from build123d import *

# Parameters (mm, degrees)
F0_R     = 2.75
F1_DEPTH = 36.8
F2_R     = 3.2
F2_R_2   = 12.15
F3_DEPTH = 12.5
F4_W     = 7
F4_H     = 7
F5_DEPTH = 25


with BuildPart() as f1:
    # F0 (on Top) → F1 (new body)
    with BuildSketch(Plane.XY):
        with BuildLine():
            ThreePointArc((-11.5987953556, -1.3), (-11.4499860347, -0.657556004), (-11.4, 0))
            ThreePointArc((-11.4, 0), (-11.4499860347, 0.657556004), (-11.5987953556, 1.3))
            Line((-11.5987953556, 1.3), (-13, 1.3))
            Line((-13, 1.3), (-13, 0))
            Line((-13, 0), (-13, -1.3))
            Line((-13, -1.3), (-11.5987953556, -1.3))
        make_face()
        with BuildLine():
            ThreePointArc((-11.5987953556, 1.3), (-11.4499860347, 0.657556004), (-11.4, 0))
            ThreePointArc((-11.4, 0), (-11.4499860347, -0.657556004), (-11.5987953556, -1.3))
            Line((-11.5987953556, -1.3), (11.5987953556, -1.3))
            ThreePointArc((11.5987953556, -1.3), (11.4, 0), (11.5987953556, 1.3))
            Line((11.5987953556, 1.3), (-11.5987953556, 1.3))
        make_face()
        with BuildLine():
            Line((-13, 1.3), (-11.5987953556, 1.3))
            ThreePointArc((-11.5987953556, 1.3), (-20.1, 0), (-11.5987953556, -1.3))
            Line((-11.5987953556, -1.3), (-13, -1.3))
            Line((-13, -1.3), (-13, 0))
            Line((-13, 0), (-13, 1.3))
        make_face()
        with Locations((-15.75, 0)):
            Circle(F0_R, mode=Mode.SUBTRACT)
        with BuildLine():
            Line((13, 1.3), (11.5987953556, 1.3))
            ThreePointArc((11.5987953556, 1.3), (11.4, 0), (11.5987953556, -1.3))
            Line((11.5987953556, -1.3), (13, -1.3))
            Line((13, -1.3), (13, 0))
            Line((13, 0), (13, 1.3))
        make_face()
        with BuildLine():
            ThreePointArc((20.1, 0), (16.407556004, 4.3000139653), (11.5987953556, 1.3))
            Line((11.5987953556, 1.3), (13, 1.3))
            Line((13, 1.3), (13, 0))
            Line((13, 0), (13, -1.3))
            Line((13, -1.3), (11.5987953556, -1.3))
            ThreePointArc((11.5987953556, -1.3), (16.407556004, -4.3000139653), (20.1, 0))
        make_face()
        with BuildLine():
            ThreePointArc((18.5, 0), (15.75, -2.75), (13, 0))
            ThreePointArc((13, 0), (15.75, 2.75), (18.5, 0))
        make_face(mode=Mode.SUBTRACT)
    extrude(amount=F1_DEPTH)

    # F2 (on Front) → F3 (cut, symmetric)
    with BuildSketch(Plane.XZ):
        with Locations((0, 18.4)):
            Circle(F2_R)
        Circle(F2_R_2)
        with Locations((0, 36.8)):
            Circle(F2_R_2)
    extrude(amount=F3_DEPTH, both=True, mode=Mode.SUBTRACT)

    # F4 (on Front) → F5 (cut)
    with BuildSketch(Plane.XZ):
        with Locations((0, 18.4)):
            Rectangle(F4_W, F4_H)
    extrude(amount=-F5_DEPTH, mode=Mode.SUBTRACT)


solid = f1.part
Geometry check sheet. Reference: the model listing, model coordinates, mm. A direction names the side the tool comes from. Coordinates: 2 decimals unless noted, no trailing zeros. Order: outer loops, then holes, each group sorted by start corner. A loop starts at its lowest first (then second) coordinate and runs counter-clockwise, first axis right, second up. Notation, with made-up numbers: (49.25, -16.75) -> (103.25, -16.75) arc R17 ccw to (103.25, -7.75) -> close; hole circle Ø7 at (67, -19). An arc over 180 degrees is marked (long way). Use a Markdown table: item, result. Add a question column.
1. Cross-section at D-D (x = 0). Enter the section's corners in (y, z), and give its area (3 significant figures).
2. Cross-section at C-C (y = -3.5). Enter the section's corners in (x, z).
3. Material ranges on L1, parallel to X at y = 0.25, z = 15.5; L2, parallel to Y at x = -15.75, z = 26; L3, parallel to X at y = -1.25, z = 33, recorded low to high.
4. Mould release check, pull along Y, two halves, no side actions. Record for faces 4 (the face through (0, -1.3, 15)), 5 (the face through (-20.097, 0.173, 18.142)), 6 (the face through (-18.5, 0.1, 18.1)), 7 (the face through (-3.5, 1, 18)): pulls with the +Y half, pulls with the -Y half, needs draft (parallel to the pull), parting line crosses it, or undercut.
5. Set-up check for faces 1 (the face through (0, 1, 21.9)), 2 (the face through (-5, 1.3, 18)), 3 (the face through (-0.267, -0.034, 24.653)): record each of +Z, -Z, +X, -X, +Y, -Y from which the full face is reachable in a straight line by a thin tool's end or side.
6. Go/stop test with flat-tipped pins: pin 1 Ø5 at (x, y) = (-7.5, 1.5) entering from -Z; pin 2 Ø0.6 at (x, y) = (0, 1) entering from -Z; pin 3 Ø1 at (x, z) = (9.5, 14.5) entering from -Y. Record where each tip stops, or that it passes through.
7. Cross-section at A-A (z = 18.4). Enter the section's corners in (x, y).
8. Cross-section at B-B (x = -15.75). Enter the section's corners in (y, z), and give its area (3 significant figures).
Filled sheet:
| question | item | result |
|---|---|---|
| 1 | outline | (-1.3, 12.15) -> (1.3, 12.15) -> (1.3, 14.9) -> (0, 14.9) -> (0, 15.2) -> (-1.3, 15.2) -> close; (-1.3, 21.6) -> (0, 21.6) -> (0, 21.9) -> (1.3, 21.9) -> (1.3, 24.65) -> (-1.3, 24.65) -> close |
| 1 | area | 15.1 mm2 |
| 2 | outline | (-18.33, 0) -> (-13.17, 0) -> (-13.17, 36.8) -> (-18.33, 36.8) -> close; (13.17, 0) -> (18.33, 0) -> (18.33, 36.8) -> (13.17, 36.8) -> close |
| 3 | L1 | -20.09 to -18.49, -13.01 to -3.5, 3.5 to 13.01, 18.49 to 20.09 |
| 3 | L2 | -4.35 to -2.75, 2.75 to 4.35 |
| 3 | L3 | -19.92 to -18.2, -13.3 to -11.54, 11.54 to 13.3, 18.2 to 19.92 |
| 4 | face 4 | pulls with the -Y half |
| 4 | face 5 | parting line crosses it |
| 4 | face 6 | undercut |
| 4 | face 7 | needs draft |
| 5 | face 1 | +Y |
| 5 | face 2 | +Z, -Z, +Y |
| 5 | face 3 | +Z, +Y, -Y |
| 6 | pin 1 | z = 6.91 |
| 6 | pin 2 | z = 12.15 |
| 6 | pin 3 | y = -1.3 |
| 7 | outline | (-11.6, -1.3) -> (-3.2, -1.3) -> (-3.2, 0) -> (-3.5, 0) -> (-3.5, 1.3) -> (-11.6, 1.3) arc R4.35 ccw (long way) to start; (3.2, -1.3) -> (11.6, -1.3) arc R4.35 ccw (long way) to (11.6, 1.3) -> (3.5, 1.3) -> (3.5, 0) -> (3.2, 0) -> close; hole circle Ø5.5 at (-15.75, 0); hole circle Ø5.5 at (15.75, 0) |
| 8 | outline | (-4.35, 0) -> (-2.75, 0) -> (-2.75, 36.8) -> (-4.35, 36.8) -> close; (2.75, 0) -> (4.35, 0) -> (4.35, 36.8) -> (2.75, 36.8) -> close |
| 8 | area | 118 mm2 |
